```python
from build123d import *

# Parameters (mm, degrees)
F0_R     = 12.7
F0_R_2   = 44.45
F1_DEPTH = 3.175


# Not quite as in the source:
# - a feature names something its author has since deleted; it is built from what else it names


with BuildPart() as f1:
    # F0 (on Top) → F1 (new body, symmetric)
    with BuildSketch(Plane.XY):
        with BuildLine():
            ThreePointArc((46.9318292839, -42.7744479808), (59.0683155093, -34.6129457767), (73.3853173936, -31.624991096))
            ThreePointArc((73.3853173936, -31.624991096), (75.1406474031, -31.6432934166), (76.8932712405, -31.7424301998))
            ThreePointArc((76.8932712405, -31.7424301998), (107.95, 0), (76.8932712405, 31.7424301998))
            ThreePointArc((76.8932712405, 31.7424301998), (75.1406474031, 31.6432934166), (73.3853173936, 31.624991096))
            ThreePointArc((73.3853173936, 31.624991096), (59.0683155093, 34.6129457767), (46.9318292839, 42.7744479808))
            ThreePointArc((46.9318292839, 42.7744479808), (0, 63.5), (-46.9318292839, 42.7744479808))
            ThreePointArc((-46.9318292839, 42.7744479808), (-60.7012108245, 33.968607894), (-76.8932712405, 31.7424301998))
            ThreePointArc((-76.8932712405, 31.7424301998), (-107.95, 0), (-76.8932712405, -31.7424301998))
            ThreePointArc((-76.8932712405, -31.7424301998), (-60.7012108245, -33.968607894), (-46.9318292839, -42.7744479808))
            ThreePointArc((-46.9318292839, -42.7744479808), (0, -63.5), (46.9318292839, -42.7744479808))
        make_face()
        with Locations((-76.2, 0)):
            Circle(F0_R, mode=Mode.SUBTRACT)
        Circle(F0_R_2, mode=Mode.SUBTRACT)
        with Locations((76.2, 0)):
            Circle(F0_R, mode=Mode.SUBTRACT)
    extrude(amount=F1_DEPTH, both=True)


solid = f1.part
```
Build history of the part. All positions in model axes, mm. Give positions to 0.01 mm unless a question says otherwise; leave off trailing zeros. Loops run counter-clockwise (first coordinate to the right, second up) from the corner with the lowest first, then second, coordinate; pieces in that order, holes last. Notation, with made-up numbers: (86, 39.25) -> (128, 39.25) arc R27 cw to (128, 62.25) -> close; hole circle Ø8 at (25, 69.25). An arc over 180 degrees is marked (long way). One line per question, with ' | ' between items. Start each with the question number.
1) Cut at B-B (z = 0). Give the cut face in (x, y).
2) Two-plate mould, pull along X, no slides. Class faces 1 (the flat face through (46, 1, -3.175)), 2 (the cylindrical face through (0.739, 63.496, 0.044)), 3 (the cylindrical face through (-64.086, 3.815, -0.044)): released by +X, released by -X, zero draft, split by the parting line, or undercut.
3) Cut at D-D (x = -24.5). Give the cut face in (y, z) (3 decimals), plus the area to 3 significant figures.
4) Cut at A-A (x = 0). Give the cut face in (y, z) (3 decimals).
5) Probe L1, parallel to Y at x = 76.2, z = -1.5; L2, parallel to X at y = -40, z = -2.25; L3, parallel to Y at x = 4, z = -2.75. List the from-to ranges inside material, lowest first.
6) Cut at C-C (y = 0). Give the cut face in (x, z) (3 decimals).
7) Pin check, flat tip, straight feed: pin 1 (3 mm diameter, centred on y = -20.5, z = -1, fed in from -X). Stop position of the tip, or through.
Return value:
1) outline: (-76.89, -31.74) arc R38.1 cw to (-46.93, -42.77) arc R63.5 ccw to (46.93, -42.77) arc R38.1 cw to (76.89, -31.74) arc R31.75 ccw to (76.89, 31.74) arc R38.1 cw to (46.93, 42.77) arc R63.5 ccw to (-46.93, 42.77) arc R38.1 cw to (-76.89, 31.74) arc R31.75 ccw to start; hole circle Ø25.4 at (-76.2, 0); hole circle Ø88.9 at (0, 0); hole circle Ø25.4 at (76.2, 0)
2) face 1: zero draft | face 2: split by the parting line | face 3: undercut
3) outline: (-58.583, -3.175) -> (-37.088, -3.175) -> (-37.088, 3.175) -> (-58.583, 3.175) -> close; (37.088, -3.175) -> (58.583, -3.175) -> (58.583, 3.175) -> (37.088, 3.175) -> close | area: 273 mm^2
4) outline: (-63.5, -3.175) -> (-44.45, -3.175) -> (-44.45, 3.175) -> (-63.5, 3.175) -> close; (44.45, -3.175) -> (63.5, -3.175) -> (63.5, 3.175) -> (44.45, 3.175) -> close
5) L1: -31.69 to -12.7, 12.7 to 31.69 | L2: -50.03 to -19.39, 19.39 to 50.03 | L3: -63.37 to -44.27, 44.27 to 63.37
6) outline: (-107.95, -3.175) -> (-88.9, -3.175) -> (-88.9, 3.175) -> (-107.95, 3.175) -> close; (-63.5, -3.175) -> (-44.45, -3.175) -> (-44.45, 3.175) -> (-63.5, 3.175) -> close; (44.45, -3.175) -> (63.5, -3.175) -> (63.5, 3.175) -> (44.45, 3.175) -> close; (88.9, -3.175) -> (107.95, -3.175) -> (107.95, 3.175) -> (88.9, 3.175) -> close
7) pin 1: x = -101.64
